```python
from build123d import *

# Parameters (mm, degrees)
BOSS_EXTRUDE1_DEPTH = 10.16
CUT_EXTRUDE1_DEPTH  = 21.32
SKETCH3_R           = 3.302
CUT_EXTRUDE2_DEPTH  = 16.24
SKETCH4_W           = 15.24
SKETCH4_H           = 10.16
BOSS_EXTRUDE2_DEPTH = 5.08


with BuildPart() as part:
    # Sketch1 → Boss-Extrude1 (new body, symmetric)
    with BuildSketch(Plane(origin=(0, 0, 0), x_dir=(0, 0, -1), z_dir=(1, 0, 0))):
        with BuildLine():
            Line((54.313848142, 17.78), (62.23, 17.78))
            Line((62.23, 17.78), (62.23, 30.48))
            Line((62.23, 30.48), (72.39, 30.48))
            Line((72.39, 30.48), (72.39, 17.78))
            Line((72.39, 17.78), (123.19, 17.78))
            Line((123.19, 17.78), (123.19, 38.1))
            Line((123.19, 38.1), (138.43, 38.1))
            Line((138.43, 38.1), (138.43, -38.1))
            Line((138.43, -38.1), (123.19, -38.1))
            Line((123.19, -38.1), (123.19, -17.78))
            Line((123.19, -17.78), (72.39, -17.78))
            Line((72.39, -17.78), (72.39, -30.48))
            Line((72.39, -30.48), (62.23, -30.48))
            Line((62.23, -30.48), (62.23, -17.78))
            Line((62.23, -17.78), (54.313848142, -17.78))
            ThreePointArc((54.313848142, -17.78), (57.15, 0), (54.313848142, 17.78))
        make_face()
    extrude(amount=BOSS_EXTRUDE1_DEPTH, both=True)

    # Sketch2 → Cut-Extrude1 (cut, through all)
    with BuildSketch(Plane(origin=(10.16, 0, 0), x_dir=(0, 0, -1), z_dir=(1, 0, 0))):
        with BuildLine():
            Line((72.39, 9.91925318), (72.39, -9.91925318))
            ThreePointArc((72.39, -9.91925318), (73.040490814, -11.02790478), (74.325603731, -11.000859243))
            Line((74.325603731, -11.000859243), (90.444390149, -1.081606062))
            ThreePointArc((90.444390149, -1.081606062), (91.048786418, 0), (90.444390149, 1.081606062))
            Line((90.444390149, 1.081606062), (74.325603731, 11.000859243))
            ThreePointArc((74.325603731, 11.000859243), (73.040490814, 11.02790478), (72.39, 9.91925318))
        make_face()
        with BuildLine():
            Line((123.19, 9.91925318), (123.19, -9.91925318))
            ThreePointArc((123.19, -9.91925318), (122.539509186, -11.02790478), (121.254396269, -11.000859243))
            Line((121.254396269, -11.000859243), (105.135609851, -1.081606062))
            ThreePointArc((105.135609851, -1.081606062), (104.531213582, 0), (105.135609851, 1.081606062))
            Line((105.135609851, 1.081606062), (121.254396269, 11.000859243))
            ThreePointArc((121.254396269, 11.000859243), (122.539509186, 11.02790478), (123.19, 9.91925318))
        make_face()
        with BuildLine():
            Line((86.873499611, 9.840393938), (97.124396269, 3.53214984))
            ThreePointArc((97.124396269, 3.53214984), (97.79, 3.343755902), (98.455603731, 3.53214984))
            Line((98.455603731, 3.53214984), (108.706500389, 9.840393938))
            ThreePointArc((108.706500389, 9.840393938), (109.262890869, 11.267875918), (108.040896659, 12.192))
            Line((108.040896659, 12.192), (87.539103341, 12.192))
            ThreePointArc((87.539103341, 12.192), (86.317109131, 11.267875918), (86.873499611, 9.840393938))
        make_face()
        with BuildLine():
            Line((87.539103341, -12.192), (108.040896659, -12.192))
            ThreePointArc((108.040896659, -12.192), (109.262890869, -11.267875918), (108.706500389, -9.840393938))
            Line((108.706500389, -9.840393938), (98.455603731, -3.53214984))
            ThreePointArc((98.455603731, -3.53214984), (97.79, -3.343755902), (97.124396269, -3.53214984))
            Line((97.124396269, -3.53214984), (86.873499611, -9.840393938))
            ThreePointArc((86.873499611, -9.840393938), (86.317109131, -11.267875918), (87.539103341, -12.192))
        make_face()
    extrude(amount=-CUT_EXTRUDE1_DEPTH, mode=Mode.SUBTRACT)

    # Sketch3 → Cut-Extrude2 (cut, through all)
    with BuildSketch(Plane.XY.offset(-123.19)):
        with Locations((0, 27.94)):
            Circle(SKETCH3_R)
        with Locations((0, -27.94)):
            Circle(SKETCH3_R)
    extrude(amount=-CUT_EXTRUDE2_DEPTH, mode=Mode.SUBTRACT)

    # Sketch4 → Boss-Extrude2 (add)
    with BuildSketch(Plane(origin=(10.16, 0, 0), x_dir=(0, 0, -1), z_dir=(1, 0, 0))):
        with Locations((130.81, 0)):
            Rectangle(SKETCH4_W, SKETCH4_H)
    extrude(amount=BOSS_EXTRUDE2_DEPTH)


solid = part.part
```
Here's how the part is built. I have some questions about the finished solid (model axes, mm). A direction names the side the tool comes from. Coordinates: 2 decimals unless noted, no trailing zeros. Order: outer loops, then holes, each group sorted by start corner. A loop starts at its lowest first (then second) coordinate and runs counter-clockwise, first axis right, second up.
Item 1: If we section it at C-C, the plane z = -70: List the corners of the cut face in (x, y) for me.
Response values:
outline: (-10.16, -30.48) - (10.16, -30.48) - (10.16, 30.48) - (-10.16, 30.48) - close
Item 2: If we section it at A-A, the plane x = 0: Give the number of separate pieces and of enclosed holes in the cut face, then the cut area to 3 significant figures.
Response values:
separate pieces: 3
enclosed holes: 4
area: 2,870 mm2
Item 3: I need wall thicknesses on probe 1 along Y at (x, z) = (0, -134.5); probe 2 along Z at (x, y) = (-3, 26); probe 3 along Z at (x, y) = (10, -10). Which ranges of each line are inside material? Lowest first, please.
Response values:
probe 1: y = -38.1 to -31.24, -24.64 to 24.64, 31.24 to 38.1
probe 2: z = -138.43 to -123.19, -72.39 to -62.23
probe 3: z = -138.43 to -123.19, -119.63 to -108.91, -86.67 to -75.95, -72.39 to -56.27
Item 4: If we section it at D-D, the plane x = 11.25: List the corners of the cut face in (y, z) for me.
Response values:
outline: (-5.08, -138.43) - (5.08, -138.43) - (5.08, -123.19) - (-5.08, -123.19) - close
Item 5: If we section it at B-B, the plane y = -27.94: List the corners of the cut face in (x, z) for me, then the cut area to 3 significant figures.
Response values:
outline: (-10.16, -138.43) - (-3.3, -138.43) - (-3.3, -123.19) - (-10.16, -123.19) - close; (-10.16, -72.39) - (10.16, -72.39) - (10.16, -62.23) - (-10.16, -62.23) - close; (3.3, -138.43) - (10.16, -138.43) - (10.16, -123.19) - (3.3, -123.19) - close
area: 415 mm2
Item 6: Which directions (+Z, -Z, +X, -X, +Y, -Y) give clear straight access to the entire face, cutting with the end or side of a thin tool? Please do faces 3 (the face through (0.142, -11.019, -73.024)), 4 (the face through (0, 23, -123.19)), 5 (the face through (0, -30.48, -67)).
Response values:
face 3: +X, -X
face 4: +X, -X, +Y
face 5: +Z, +X, -X, -Y
Item 7: Thinking about a two-plate mould opening in X: for faces 1 (the face through (0, -24, -72.39)), 2 (the face through (-0.43, -24.666, -130.703)), which applies, pulls with the +X half, pulls with the -X half, needs draft (parallel to the pull), parting line crosses it, or undercut?
Response values:
face 1: needs draft
face 2: undercut
Item 8: I'm going to push flat-ended pins straight in: pin 1 Ø10 at (x, z) = (-3.5, -107.5) entering from -Y; pin 2 Ø8 at (x, z) = (3, -65) entering from +Y; pin 3 Ø2.5 at (x, z) = (3, -57) entering from +Y; pin 4 Ø12 at (x, y) = (12, 16) entering from -Z. Where does each tip first touch, or does it pass through?
Response values:
pin 1: stops at y = -17.78
pin 2: stops at y = 30.48
pin 3: stops at y = 17.78
pin 4: stops at z = -138.43
